For this review, use the dimensioned drawing (mm, ordinates from the lowest corner) and the shaded views. A direction names the side the tool comes from. Give positions to 0.01 mm unless a question says otherwise; leave off trailing zeros. Loops run counter-clockwise (first coordinate to the right, second up) from the corner with the lowest first, then second, coordinate; pieces in that order, holes last. Notation, with made-up numbers: M 39,9 L 86,9 A18 ccw 86,23 Z; hole C -5,-4.5 d9. An arc over 180 degrees is marked long. Use CSV: the item, a comma, the result in double quotes. Start each with the question number.
1. Take a section at A-A, the plane x = 26.25. Write out the cut boundary in (y, z), and give its area (3 significant figures).
2. Tool access review of the marked faces 1 and 2: name each direction out of +Z, -Z, +X, -X, +Y, -Y from which nothing blocks a thin tool from reaching the whole face with its end or side.
3. Take a section at D-D, the plane y = 1.5. Write out the cut boundary in (x, z), and give its area (3 significant figures).
4. Insertion check: P1, Ø1, axis at x = 3.5, z = 8.5, coming from the +Y side; P2, Ø0.5, axis at y = 0.5, z = 7, coming from the +X side; P3, Ø1.5, axis at x = 19, z = 5.5, coming from the +Y side; P4, Ø5, axis at y = 8, z = 2.5, coming from the +X side. Each pin has a flat end and moves straight along its axis. Give the tip position at first contact, or say it passes through.
5. Take a section at B-B, the plane x = 4. Write out the cut boundary in (y, z).
6. Take a section at C-C, the plane z = 8. Write out the cut boundary in (x, y), and give its area (3 significant figures).
7. To check wall thickness, follow line 1 (X direction, y = 6.5, z = 8); line 2 (Z direction, x = 4, y = 5.5); line 3 (X direction, y = 6.75, z = 8.75). State the ranges of each line that lie inside material, in increasing order. Write a range as [from, to].
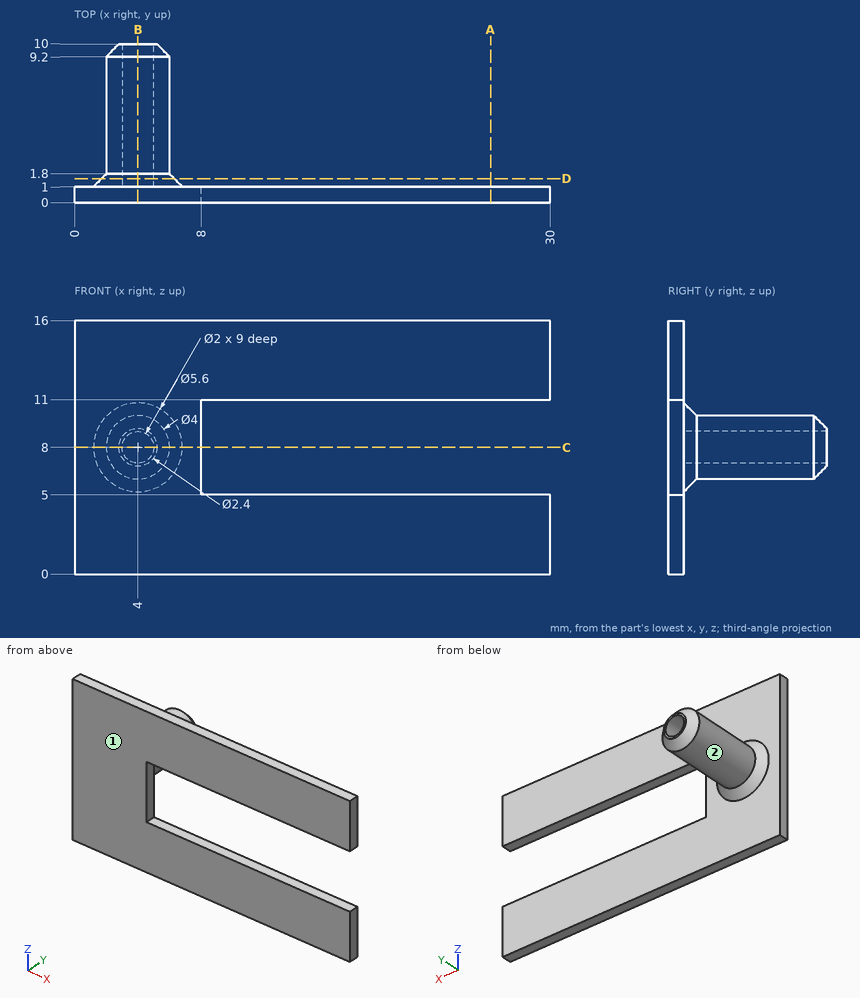
Result set:
1,outline,"M 0,0 L 1,0 L 1,5 L 0,5 Z; M 0,11 L 1,11 L 1,16 L 0,16 Z"
1,area,"10.0 mm2"
2,face 1,"+Z, -Z, +X, -X, -Y"
2,face 2,"+Y"
3,outline,"C 4,8 d4.6; hole C 4,8 d2"
3,area,"13.5 mm2"
4,P1,"y = 10"
4,P2,"x = 8"
4,P3,"y = 1"
4,P4,"through"
5,outline,"M 0,0 L 1,0 L 1,5.2 L 1.8,6 L 9.2,6 L 10,6.8 L 10,7 L 1,7 L 1,9 L 10,9 L 10,9.2 L 9.2,10 L 1.8,10 L 1,10.8 L 1,16 L 0,16 Z"
6,outline,"M 0,0 L 8,0 L 8,1 L 6.8,1 L 6,1.8 L 6,9.2 L 5.2,10 L 5,10 L 5,1 L 3,1 L 3,10 L 2.8,10 L 2,9.2 L 2,1.8 L 1.2,1 L 0,1 Z"
6,area,"26.0 mm2"
7,line 1,"[2, 3], [5, 6]"
7,line 2,"[6, 7], [9, 10]"
7,line 3,"[2.15, 3.34], [4.66, 5.85]"
